Read the model definition and answer for the solid it produces. Units are mm, in the model's axes. A direction names the side the tool comes from. Round coordinates to 2 decimals unless told otherwise and drop trailing zeros. Use one line per item in the form item = value. Start each with the question number.
1) Consider line 1 along Z through (x, y) = (23.5, 1.5); line 2 along X through (y, z) = (-2.5, -3); line 3 along X through (y, z) = (0.5, 1.75). Determine where each line is inside the solid, lowest interval first. Write a range as from..to.
2) For faces 1 (the face through (15.66, -0.54, -2.44)), 2 (the face through (1.553, 3.448, 2.028)), determine the directions among +Z, -Z, +X, -X, +Y, -Y from which every point of the face is accessible in a straight line to the end or side of a thin tool.
3) Each of these flat-tipped pins is pushed along its axis until it touches: pin 1 (0.9 mm diameter, centred on y = -4, z = -1, fed in from +X); pin 2 (1.5 mm diameter, centred on x = 4.5, y = -2, fed in from +Z); pin 3 (4 mm diameter, centred on x = 38, z = -1, fed in from -Y). Where does it stop, or does it pass through?
from build123d import *

# Parameters (mm, degrees)
BASEHEAD_DEPTH     = 3.65
INDENT_START       = -0.45625
INDENT_2_OUTLINE_R = 3.5
INDENT_2_DEPTH     = 0.45625
SKETCH4_W          = 0.5
SKETCH4_H          = 10.618802154
THDSCHPAT_COUNT    = 20
THDSCHPAT_PITCH    = 0.8


# Read off the part's stored shape, not the designer's step: Indent
with BuildPart() as part:
    # Sketch1 → BaseHead (new body)
    with BuildSketch(Plane(origin=(0, 0, 0), x_dir=(0, 0, -1), z_dir=(1, 0, 0))):
        Polygon((4, 2.309401077), (4, -2.309401077), (0, -4.618802154), (-4, -2.309401077), (-4, 2.309401077), (0, 4.618802154), align=None)
    extrude(amount=BASEHEAD_DEPTH)

    # Indent outline → Indent (revolve)
    with BuildSketch(Plane.YX):
        Polygon((2.5, 3.65), (2.5, 43.205), (2.055, 43.65), (0, 43.65), (0, 3.65), align=None)
    revolve(axis=Axis((0, 0, 0), (1, 0, 0)))

    # Indent 2 outline → Indent 2 (cut)
    with BuildSketch(Plane.ZY.offset(INDENT_START)):
        with Locations((0.033212245, 0.192376607)):
            Circle(INDENT_2_OUTLINE_R)
    extrude(amount=INDENT_2_DEPTH, mode=Mode.SUBTRACT)

    # Sketch3 → HeadChamfer (revolve, cut)
    with BuildSketch(Plane.XY, mode=Mode.PRIVATE) as headchamfer_sk:
        Polygon((0, 4), (3.244016936, 9.618802154), (3.244016936, 14.618802154), (-10, 14.618802154), (-10, 4), align=None)
    revolve(headchamfer_sk.sketch.rotate(Axis((0, 0, 0), (1, 0, 0)), 90), axis=Axis((0, 0, 0), (1, 0, 0)), mode=Mode.SUBTRACT)

    # Sketch4 → BearingFace (revolve, cut)
    with BuildSketch(Plane.XY, mode=Mode.PRIVATE) as bearingface_sk:
        with Locations((3.4, 9.309401077)):
            Rectangle(SKETCH4_W, SKETCH4_H)
    revolve(bearingface_sk.sketch.rotate(Axis((0, 0, 0), (1, 0, 0)), 90), axis=Axis((0, 0, 0), (1, 0, 0)), mode=Mode.SUBTRACT)

    # ThdSchSke → ThreadSchematic (revolve, cut)
    with BuildSketch(Plane.XY):
        Polygon((27.65, -2.055), (27.338407645, -2.5), (27.338407645, -3.125), (27.961592355, -3.125), (27.961592355, -2.5), align=None)
    threadschematic = revolve(axis=Axis((-3.175, 0, 0), (1, 0, 0)), mode=Mode.SUBTRACT)

    # ThdSchPat: ThreadSchematic ×20
    with Locations(*[(i * THDSCHPAT_PITCH, 0, 0) for i in range(1, THDSCHPAT_COUNT)]):
        add(threadschematic, mode=Mode.SUBTRACT)


solid = part.part
Geometry results:
q1.line_1 = -2..2
q1.line_2 = 0..3.65
q1.line_3 = 0.46..43.65
q2.face_1 = +X
q2.face_2 = +Z, +X, -X, +Y
q3.pin_1 = 3.65
q3.pin_2 = 2.17
q3.pin_3 = -2.5
